The drawing under review shows one solid part. Ordinate dimensions are in mm from its lowest x, y, z. A direction names the side the tool comes from. Coordinates: 2 decimals unless noted, no trailing zeros. Write each loop counter-clockwise with the first axis right and the second up, starting at its lowest first coordinate (ties: lowest second). Pieces come first, ordered by that corner, then holes.
Q1. Add section B-B, the plane z = 7.5. Give the boundary of the cut face in (x, y).
Q2. Add section A-A, the plane x = 35. Give the boundary of the cut face in (y, z), plus the area to 3 significant figures.
Q3. Add section C-C, the plane y = 35. Give the number of separate pieces and of enclosed holes in the cut face, plus the area to 3 significant figures.
Q4. Add section D-D, the plane z = 3.5. Give the boundary of the cut face in (x, y).
Q5. Clearance check with flat-ended pins moving along their axes: pin 1 Ø4 at (y, z) = (9, 8.5) entering from +X; pin 2 Ø8 at (x, y) = (50, 35) entering from +Z; pin 3 Ø5 at (x, z) = (27, 5) entering from +Y; pin 4 Ø1.5 at (y, z) = (39, 7.5) entering from +X. State where each tip first meets the part, or that it passes through.
Q6. To check wall thickness, follow probe 1 along Z at (x, y) = (56.5, 35); probe 2 along Y at (x, z) = (32.5, 7); probe 3 along Y at (x, z) = (20, 7.1). State the ranges of each line that lie inside material, in increasing order.
Q7. The part is to be moulded in two halves that separate along Y. For the marked faces 1, 2 and 3, say which applies: +Y half, -Y half, draft (parallel to the pull), parting line (faces both ways), or undercut.
Q8. Machinability: for the marked faces 4 and 5, which of the approach directions +Z, -Z, +X, -X, +Y, -Y give a long, thin tool a straight path to every point of the face, cutting with its end or side? Answer none if there is none.
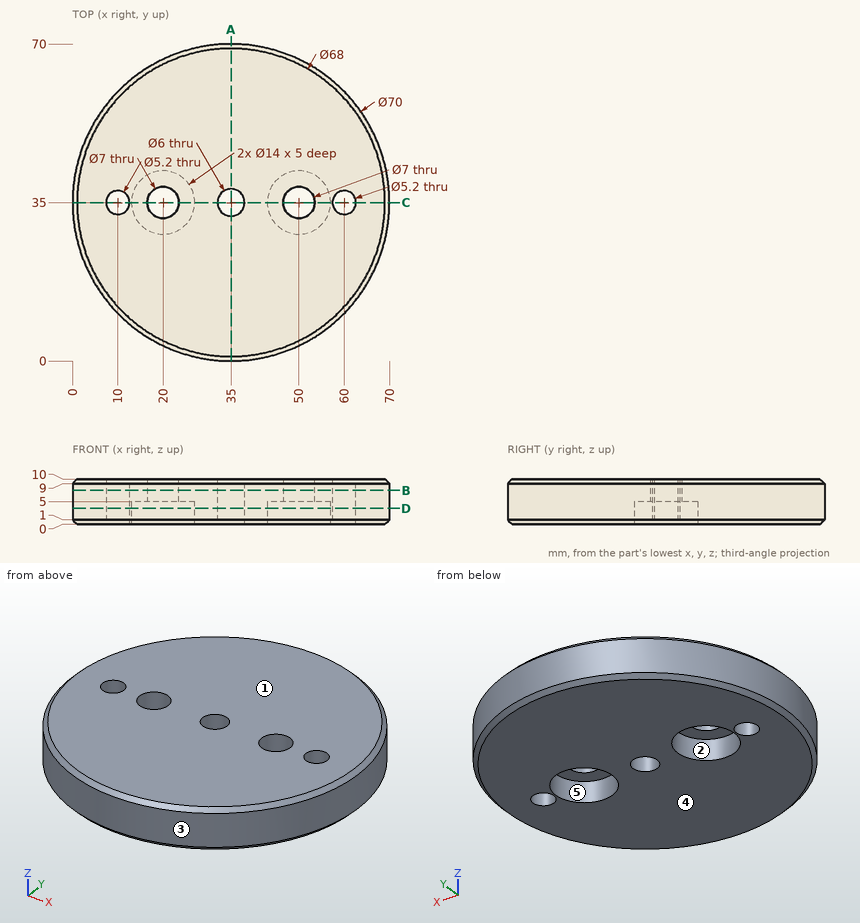
Here are the results:
1. outline: circle Ø70 at (35, 35); hole circle Ø5.2 at (10, 35); hole circle Ø7 at (20, 35); hole circle Ø6 at (35, 35); hole circle Ø7 at (50, 35); hole circle Ø5.2 at (60, 35)
2. outline: (0, 1) - (1, 0) - (32, 0) - (32, 10) - (1, 10) - (0, 9) - close; (38, 0) - (69, 0) - (70, 1) - (70, 9) - (69, 10) - (38, 10) - close
2. area: 638 mm2
3. separate pieces: 6
3. enclosed holes: 0
3. area: 324 mm2
4. outline: circle Ø70 at (35, 35); hole circle Ø5.2 at (10, 35); hole circle Ø14 at (20, 35); hole circle Ø6 at (35, 35); hole circle Ø14 at (50, 35); hole circle Ø5.2 at (60, 35)
5. pin 1: stops at x = 60.48
5. pin 2: stops at z = 10
5. pin 3: stops at y = 69.57
5. pin 4: stops at x = 69.85
6. probe 1: z = 5 to 10
6. probe 2: y = 0.09 to 33.34, 36.66 to 69.91
6. probe 3: y = 3.38 to 31.5, 38.5 to 66.62
7. face 1: draft
7. face 2: undercut
7. face 3: parting line
8. face 4: -Z, +X, -X, +Y, -Y
8. face 5: -Z
